Autodesk Inventor part; units mm, degrees
ref_plane "YZ Plane" through (0, 0, 0) normal (1, 0, 0) x (0, 1, 0)
ref_plane "XZ Plane" through (0, 0, 0) normal (0, 1, 0) x (-1, 0, 0)
ref_plane "XY Plane" through (0, 0, 0) normal (0, 0, 1) x (1, 0, 0)
sketch "Sketch1" plane through (0, 0, 0) normal (0, 0, 1) x (1, 0, 0)
  circle A0 centre (0, 0) radius 3.05
  line L0 (0, 30) -> (0, -30) construction
  circle A1 centre (0, 30) radius 7.5
  circle A2 centre (0, -30) radius 7.5
  line L1 (0, 30) -> (0, -30) construction
  line L2 (15, 30) -> (15, -30)
  line L3 (-15, -30) -> (-15, 30)
  arc A3 (15, 30) -> (-15, 30) centre (0, 30) ccw
  arc A4 (-15, -30) -> (15, -30) centre (0, -30) ccw
  point P0 (0, 0)
  dimension "d0" = 30
  dimension "d1" = 6.1
  dimension "d2" = 15
  dimension "d3" = 30
extrude "Extrusion1" add sketch "Sketch1" along normal blind 24
sketch "Sketch2" plane through (0, 0, 24) normal (0, 0, 1) x (1, 0, 0)
  circle A0 centre (0, -30) radius 7.5 construction
  circle A1 centre (0, 30) radius 7.5 construction
  circle A2 centre (0, 0) radius 3.05 construction
  line L0 (15, -30) -> (15, 30) construction
  arc A3 (15, 30) -> (-15, 30) centre (0, 30) ccw construction
  line L1 (-15, 30) -> (-15, -30) construction
  arc A4 (-15, -30) -> (15, -30) centre (0, -30) ccw construction
  line L2 (5, -16) -> (-5, -16)
  line L3 (-5, -16) -> (-5, 16)
  line L4 (-5, 16) -> (5, 16)
  line L5 (5, 16) -> (5, -16)
  line L6 (5, -16) -> (-5, 16) construction
  line L7 (-5, -16) -> (5, 16) construction
  dimension "d6" = 10
  dimension "d7" = 32
extrude "Extrusion2" cut sketch "Sketch2" against normal blind 14
sketch "Sketch3" plane through (15, -30, 0) normal (1, 0, 0) x (0, 0, -1)
  line L0 (0, 60) -> (0, 0) construction
  line L1 (0, 60) -> (-24, 60) construction
  line L2 (-24, 0) -> (-24, 60) construction
  line L3 (0, 0) -> (-24, 0) construction
  line L4 (-24, 14) -> (-24, 46) construction
  line L5 (-24, 14) -> (-10, 14) construction
  line L6 (-10, 14) -> (-10, 46) construction
  line L7 (-24, 46) -> (-10, 46) construction
  line L8 (-24, 30) -> (-35, 30) construction
  circle A0 centre (-35, 30) radius 2.9
  arc A1 (-42.8398, 36.2079) -> (-42.8398, 23.7921) centre (-35, 30) ccw
  line L9 (-42.8398, 36.2079) -> (-24, 60)
  line L10 (-42.8398, 23.7921) -> (-24, 0)
  line L11 (-24, 60) -> (-24, 0)
  line L12 (-24, 52.5) -> (-24, 67.5)
  point P0 (0, 30)
  dimension "d10" = 25
  dimension "d11" = 5.8
  dimension "d12" = 10
extrude "Extrusion3" add sketch "Sketch3" against normal up to surface (10 mm away)
mirror "Mirror1" about plane through (0, 0, 0) normal (1, 0, 0) of "Extrusion3"
properties part number "combo cross head"
Source: CAD feature listing. Evaluate the final solid. Frame: model axes, mm. A direction names the side the tool comes from. Round coordinates to 2 decimals unless told otherwise and drop trailing zeros. Write each loop counter-clockwise with the first axis right and the second up, starting at its lowest first coordinate (ties: lowest second). Pieces come first, ordered by that corner, then holes. Notation, with made-up numbers: M 80.5,3.5 L 126.5,3.5 A25 cw 126.5,20.5 Z; hole C 49,13 d1. An arc over 180 degrees is marked long. Answer as a JSON object with one key per item and string values. Group by question number.
(1) Section query B-B on y = 0. Output: boundary loops of the cut face in (x, z).
(2) Mould query, pull axis Y, two halves, no side actions, for faces 1 (the flat face through (10.07, -17.94, 33.55)), 2 (the flat face through (0, 19, 24)), 3 (the flat face through (3.3, 0.2, 10)). Classes: +Y half, -Y half, draft (parallel to the pull), parting line (faces both ways), or undercut.
(3) Reachability of faces 4 (the flat face through (5, 0, 24)), 5 (the cylindrical face through (-1.63, -22.68, 11.83)), 6 (the cylindrical face through (10, 0, 45)), 7 (the cylindrical face through (-10.07, -0.871, 32.234)), 8 (the flat face through (0, -19, 24)) from +Z, -Z, +X, -X, +Y, -Y: full face, straight path, thin tool, end or side. Return the list, or none.
(4) Section query C-C on z = 3. Output: boundary loops of the cut face in (x, y).
(5) Section query D-D on z = 34. Output: boundary loops of the cut face in (x, y).
(6) Section query A-A on x = 0. Output: boundary loops of the cut face in (y, z).
(7) Ray query, line 1 (Y direction, x = 0, z = 4); line 2 (Y direction, x = 0, z = 11.5); line 3 (X direction, y = 2, z = 15.5). Return the intervals inside material, ascending. Write a range as [from, to].
(8) First-contact query: pin 1 (10 mm diameter, centred on x = 1.5, z = 4.5, fed in from +Y); pin 2 (13.5 mm diameter, centred on x = 0, y = -30, fed in from -Z); pin 3 (5 mm diameter, centred on x = -5.5, z = 25, fed in from -Y); pin 4 (4 mm diameter, centred on x = -10, z = 20.5, fed in from +Y). Flat tips, straight axial feed; report the tip coordinate or a pass-through.
Computed values:
{
 "1": {"outline": "M -15,0 L -3.05,0 L -3.05,10 L -5,10 L -5,32.1 L -15,32.1 Z; M -15,37.9 L -5,37.9 L -5,45 L -15,45 Z; M 3.05,0 L 15,0 L 15,32.1 L 5,32.1 L 5,10 L 3.05,10 Z; M 5,37.9 L 15,37.9 L 15,45 L 5,45 Z"},
 "2": {"face 1": "-Y half", "face 2": "draft", "face 3": "undercut"},
 "3": {"face 4": "+Z", "face 5": "-Z", "face 6": "+Z, +X, -X", "face 7": "+X, -X", "face 8": "+Z, +Y, -Y"},
 "4": {"outline": "M -15,-30 A15 ccw 15,-30 L 15,30 A15 ccw -15,30 Z; hole C 0,-30 d15; hole C 0,30 d15; hole C 0,0 d6.1"},
 "5": {"outline": "M -15,-17.37 L -5,-17.37 L -5,-2.72 L -15,-2.72 Z; M -15,2.72 L -5,2.72 L -5,17.37 L -15,17.37 Z; M 5,-17.37 L 15,-17.37 L 15,-2.72 L 5,-2.72 Z; M 5,2.72 L 15,2.72 L 15,17.37 L 5,17.37 Z"},
 "6": {"outline": "M -45,0 L -37.5,0 L -37.5,24 L -45,24 Z; M -22.5,0 L -3.05,0 L -3.05,10 L -16,10 L -16,24 L -22.5,24 Z; M 3.05,0 L 22.5,0 L 22.5,24 L 16,24 L 16,10 L 3.05,10 Z; M 37.5,0 L 45,0 L 45,24 L 37.5,24 Z"},
 "7": {"line 1": "[-45, -37.5], [-22.5, -3.05], [3.05, 22.5], [37.5, 45]", "line 2": "[-45, -37.5], [-22.5, -16], [16, 22.5], [37.5, 45]", "line 3": "[-15, -5], [5, 15]"},
 "8": {"pin 1": "y = 45", "pin 2": "z = 24", "pin 3": "y = -44.65", "pin 4": "y = 42.69"}
}
